Build history of the part. All positions in model axes, mm. A direction names the side the tool comes from. Coordinates: 2 decimals unless noted, no trailing zeros. Loops run counter-clockwise (first coordinate to the right, second up) from the corner with the lowest first, then second, coordinate; pieces in that order, holes last.
Item 1: Cut at A-A (x = 4). List the corners of the cut face in (y, z).
Item 2: Flat gauge pins, fed straight in: pin 1 (8 mm diameter, centred on x = 11, z = 18.5, fed in from +Y); pin 2 (3 mm diameter, centred on x = 14.5, y = 30.5, fed in from +Z); pin 3 (4 mm diameter, centred on x = 7.5, y = 19, fed in from +Z); pin 4 (3 mm diameter, centred on y = 28, z = 6.5, fed in from -X). Where does each tip first touch, or does it go through?
Item 3: Cut at D-D (x = 16). List the corners of the cut face in (y, z).
Item 4: 3-axis set-ups, long thin cutter, end or side, ignore diameter. For faces 1 (the face through (15.28, 7.64, 19.35)), 2 (the face through (20, 20, 0)), 3 (the face through (16, 32, 19)): which of +Z, -Z, +X, -X, +Y, -Y reach the whole face in a straight line?
Item 5: Drill centre lines: line 1 along X through (y, z) = (7.5, 11.5); line 2 along Y through (x, z) = (13, 13); line 3 along Z through (x, y) = (6, 28) (3 decimals). Where is each one in solid material? Low to high.
Item 6: Cut at B-B (y = 34). List the corners of the cut face in (x, z).
Item 7: Cut at C-C (z = 12). List the corners of the cut face in (x, y), and give its area (3 significant figures).
from build123d import *

# Parameters (mm, degrees)
F1_DEPTH = 15
F3_DEPTH = 40.001
F4_DEPTH = 30
F8_DEPTH = 7.372541402


with BuildPart() as f1:
    # F0 (on Top) → F1 (new body)
    with BuildSketch(Plane.XY):
        Polygon((40, 20), (0, 0), (40, 0), align=None)
        Polygon((0, 40), (0, 0), (40, 20), align=None)
        Polygon((40, 40), (0, 40), (40, 20), align=None)
    extrude(amount=F1_DEPTH)

    # F2 (on face) → F3 (cut, through all)
    with BuildSketch(Plane.YZ.offset(40)):
        Polygon((0, 9), (20, 15), (0, 15), align=None)
        Polygon((40, 15), (20, 15), (40, 9), align=None)
    extrude(amount=-F3_DEPTH, mode=Mode.SUBTRACT)

    # F0 (on Top) → F4 (join)
    with BuildSketch(Plane.XY):
        Polygon((0, 40), (0, 0), (40, 20), align=None)
    extrude(amount=F4_DEPTH)

    # F7 (on 3pt) → F8 (cut, through all)
    with BuildSketch(Plane(origin=(5.4339622642, 0, 28.9811320755), x_dir=(0.9828721869, 0, -0.1842885351), z_dir=(-0.1842885351, 0, -0.9828721869))):
        Polygon((35.1683954387, -20), (-5.5286560515, 0), (-5.5286560515, -40), align=None)
    extrude(amount=-F8_DEPTH, mode=Mode.SUBTRACT)


solid = f1.part
Filled sheet:
1. outline: (0, 0) - (40, 0) - (40, 9) - (38, 9.6) - (38, 29.25) - (2, 29.25) - (2, 9.6) - (0, 9) - close
2. pin 1: stops at y = 36.5
2. pin 2: stops at z = 27.56
2. pin 3: stops at z = 28.97
2. pin 4: stops at x = 0
3. outline: (0, 0) - (40, 0) - (40, 9) - (32, 11.4) - (32, 27) - (8, 27) - (8, 11.4) - (0, 9) - close
4. face 1: +Z, +X, -Y
4. face 2: -Z, +X, -X, +Y, -Y
4. face 3: +Z, +X, +Y
5. line 1: x = 0 to 15
5. line 2: y = 6.5 to 33.5
5. line 3: z = 0 to 28.875
6. outline: (0, 0) - (40, 0) - (40, 10.8) - (12, 10.8) - (12, 27.75) - (0, 30) - close
7. outline: (0, 0) - (20, 10) - (40, 10) - (40, 30) - (20, 30) - (0, 40) - close
7. area: 1,000 mm2
